Geometry check sheet. Reference: the model listing, model coordinates, mm. A direction names the side the tool comes from. Coordinates: 2 decimals unless noted, no trailing zeros. Write each loop counter-clockwise with the first axis right and the second up, starting at its lowest first coordinate (ties: lowest second). Pieces come first, ordered by that corner, then holes. Notation, with made-up numbers: M -19,45 L -4,45 A13 cw -4,69 Z; hole C -0.75,10 d10. An arc over 180 degrees is marked long. Put each result on its own line as item: value. Start each with the question number.
1) Mould release check, pull along X, two halves, no side actions. Record for faces 1 (the cylindrical face through (12.05, -19.3, 132.07)), 2 (the flat face through (15, 53.5, 132)), 3 (the flat face through (30, 1, 99)): released by +X, released by -X, zero draft, split by the parting line, or undercut.
2) Cross-section at A-A on y = -3.5. Record the cut outline in (x, z).
3) Cross-section at C-C on x = 26.25. Record the cut outline in (y, z).
4) Cross-section at D-D on z = 32. Record the cut outline in (x, y), plus the area to 3 significant figures.
5) Cross-section at B-B on z = 10. Record the cut outline in (x, y), plus the area to 3 significant figures.
6) Gauge pin test, flat ends, axial feed: pin 1 (5 mm diameter, centred on x = 15, y = -22, fed in from +Z); pin 2 (0.9 mm diameter, centred on x = 15.5, z = 115.5, fed in from -Y); pin 3 (1.5 mm diameter, centred on x = 4.5, y = -17.5, fed in from -Z); pin 4 (2 mm diameter, centred on x = 25, z = 84.5, fed in from +Y). Record the tip position at first contact, or that the pin passes through.
7) Scan lines: line 1 along Y through (x, z) = (15, 133.5); line 2 along Z through (x, y) = (15, 8); line 3 along X through (y, z) = (5, 70). Record each from-to range of solid material in increasing order.
8) Set-up check for faces 4 (the cylindrical face through (14.479, -117.034, 132.07)), 5 (the flat face through (6, 0, 64)), 6 (the flat face through (15, 10, 63)): record each of +Z, -Z, +X, -X, +Y, -Y from which the full face is reachable in a straight line by a thin tool's end or side.
from build123d import *

# Parameters (mm, degrees)
F1_DEPTH = 30
F2_R     = 4
F3_DEPTH = 53.501
F4_R     = 4
F5_DEPTH = 137.001
F6_R     = 1.5
F7_DEPTH = 5


with BuildPart() as f1:
    # F0 (on Right) → F1 (new body)
    with BuildSketch(Plane.YZ):
        Polygon((0, 127), (0, 0), (10, 0), (10, 127), (53.5, 127), (53.5, 137), (-135, 137), (-135, 127), align=None)
    extrude(amount=F1_DEPTH)

    # F2 (on face) → F3 (cut, through all)
    with BuildSketch(Plane.XZ):
        with Locations((15, 70)):
            Circle(F2_R)
        with Locations((15, 10)):
            Circle(F2_R)
    extrude(amount=-F3_DEPTH, mode=Mode.SUBTRACT)

    # F4 (on face) → F5 (cut, through all)
    with BuildSketch(Plane.XY.offset(137)):
        with Locations((15, 45)):
            Circle(F4_R)
        with Locations((15, 30)):
            Circle(F4_R)
        with Locations((15, -3.5)):
            Circle(F4_R)
        with Locations((15, -22)):
            Circle(F4_R)
        with Locations((15, -121)):
            Circle(F4_R)
    extrude(amount=-F5_DEPTH, mode=Mode.SUBTRACT)

    # F6 (on face) → F7 (cut)
    with BuildSketch(Plane.XZ):
        with Locations((15, 110)):
            Circle(F6_R)
        with Locations((15, 115)):
            Circle(F6_R)
    extrude(amount=-F7_DEPTH, mode=Mode.SUBTRACT)


solid = f1.part
Answer key:
1. face 1: undercut
1. face 2: zero draft
1. face 3: released by +X
2. outline: M 0,127 L 11,127 L 11,137 L 0,137 Z; M 19,127 L 30,127 L 30,137 L 19,137 Z
3. outline: M -135,127 L 0,127 L 0,0 L 10,0 L 10,127 L 53.5,127 L 53.5,137 L -135,137 Z
4. outline: M 0,0 L 13.06,0 A4 cw 16.94,0 L 30,0 L 30,10 L 0,10 Z
4. area: 299 mm²
5. outline: M 0,0 L 11,0 L 11,10 L 0,10 Z; M 19,0 L 30,0 L 30,10 L 19,10 Z
5. area: 220 mm²
6. pin 1: passes through
6. pin 2: stops at y = 5
6. pin 3: stops at z = 127
6. pin 4: stops at y = 10
7. line 1: y = -135 to -125, -117 to -26, -18 to -7.5, 0.5 to 26, 34 to 41, 49 to 53.5
7. line 2: z = 0 to 6, 14 to 66, 74 to 137
7. line 3: x = 0 to 11, 19 to 30
8. face 4: +Z, -Z
8. face 5: -Z, +X, -X, -Y
8. face 6: -Z, +X, -X, +Y
